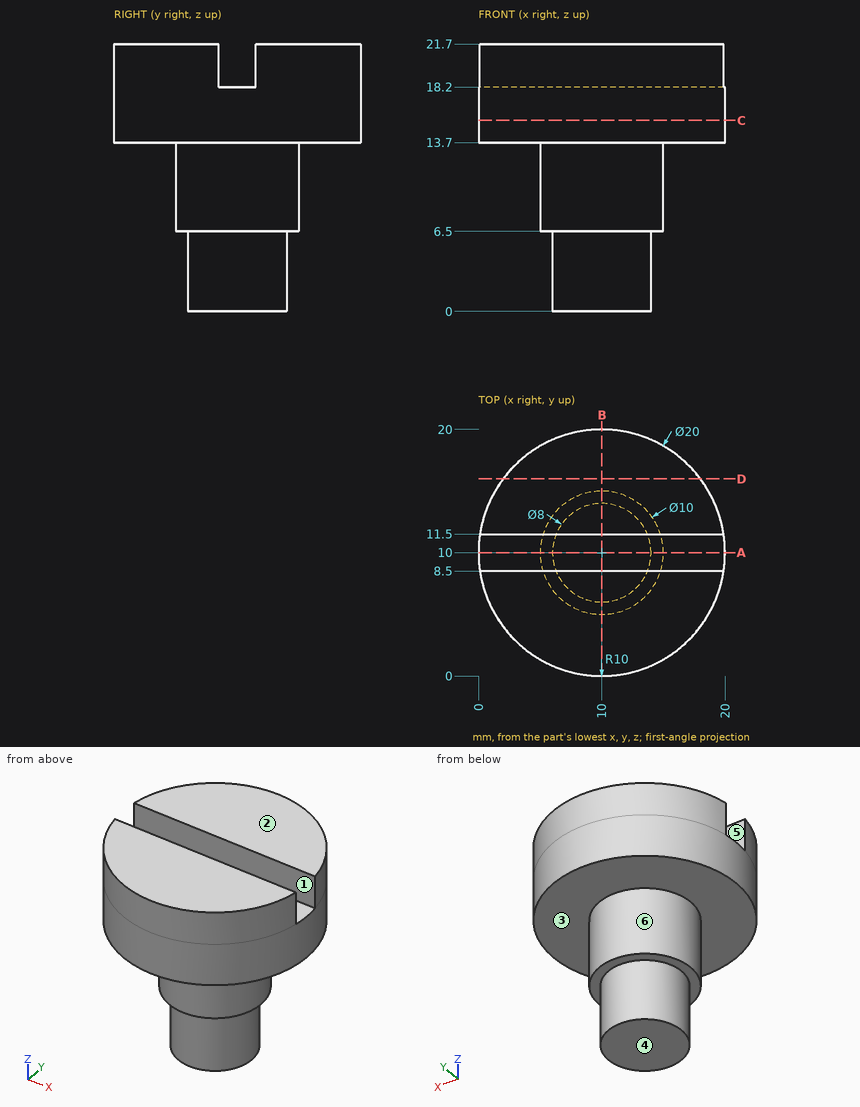
Source: three-view drawing plus pictorial views. Frame: mm from the lowest corner of the part. A direction names the side the tool comes from. Coordinates: 2 decimals unless noted, no trailing zeros. Order: outer loops, then holes, each group sorted by start corner. A loop starts at its lowest first (then second) coordinate and runs counter-clockwise, first axis right, second up.
Item 1: Pull-direction query (Y, two-part tool) for the marked faces 4, 5 and 6; classes: pulls with the +Y half, pulls with the -Y half, needs draft (parallel to the pull), parting line crosses it, or undercut.
Output values:
face 4: needs draft
face 5: undercut
face 6: parting line crosses it
Item 2: Cut plane C-C (z = 15.5). Return loops of the section in (x, y), plus the area to 3 significant figures.
Output values:
outline: circle Ø20 at (10, 10)
area: 314 mm2
Item 3: Cut plane A-A (y = 10). Return loops of the section in (x, z), plus the area to 3 significant figures.
Output values:
outline: (0, 13.7) - (5, 13.7) - (5, 6.5) - (6, 6.5) - (6, 0) - (14, 0) - (14, 6.5) - (15, 6.5) - (15, 13.7) - (20, 13.7) - (20, 18.2) - (0, 18.2) - close
area: 214 mm2
Item 4: Set-up query: the marked faces 1, 2 and 3. Return all of +Z, -Z, +X, -X, +Y, -Y with unobstructed straight access to the full face (end or side cutting, diameter ignored); none if empty.
Output values:
face 1: +Z, +X, -X
face 2: +Z, +X, -X, +Y, -Y
face 3: -Z
Item 5: First-contact query: P1, Ø3, axis at x = 5, z = 19.5, coming from the +Y side; P2, Ø12, axis at x = 2.5, z = 13.5, coming from the -Y side; P3, Ø1.8, axis at x = 8.5, z = 20.5, coming from the -Y side. Flat tips, straight axial feed; report the tip coordinate or a pass-through.
Output values:
P1: stops at y = 19.37
P2: stops at y = 0.11
P3: stops at y = 0.02
Item 6: Material intervals for line 1 (Y direction, x = 14.5, z = 19.5); line 2 (Z direction, x = 16.25, y = 15.75); line 3 (Y direction, x = 14, z = 21.25), sorted ascending.
Output values:
line 1: y = 1.07 to 8.5, 11.5 to 18.93
line 2: z = 13.7 to 21.7
line 3: y = 0.83 to 8.5, 11.5 to 19.17
Item 7: Cut plane B-B (x = 10). Return loops of the section in (y, z).
Output values:
outline: (0, 13.7) - (5, 13.7) - (5, 6.5) - (6, 6.5) - (6, 0) - (14, 0) - (14, 6.5) - (15, 6.5) - (15, 13.7) - (20, 13.7) - (20, 21.7) - (11.5, 21.7) - (11.5, 18.2) - (8.5, 18.2) - (8.5, 21.7) - (0, 21.7) - close
Item 8: Cut plane D-D (y = 16). Return loops of the section in (x, z), plus the area to 3 significant figures.
Output values:
outline: (2, 13.7) - (18, 13.7) - (18, 21.7) - (2, 21.7) - close
area: 128 mm2
